Source: CAD feature listing. Evaluate the final solid. Frame: model axes, mm. Face numbers are marked on the shaded views. A direction names the side the tool comes from. Round coordinates to 2 decimals unless told otherwise and drop trailing zeros. Loops run counter-clockwise (first coordinate to the right, second up) from the corner with the lowest first, then second, coordinate; pieces in that order, holes last. Notation, with made-up numbers: (5.5, 7.25) -> (9.5, 7.25) arc R16 cw to (9.5, 33.25) -> close; hole circle Ø8 at (28, 75.25). An arc over 180 degrees is marked (long way). Write item = value, one per line.
from build123d import *

# Parameters (mm, degrees)
F0_R     = 20.6375
F0_R_2   = 6
F1_DEPTH = 237.33125
F2_DEPTH = 263.525
F3_R     = 3.175
F4_DEPTH = 6.35


with BuildPart() as f1:
    # F0 (on Right) → F1 (new body, symmetric)
    with BuildSketch(Plane.YZ):
        Circle(F0_R)
        Circle(F0_R_2, mode=Mode.SUBTRACT)
    extrude(amount=F1_DEPTH, both=True)

    # F0 (on Right) → F2 (join, symmetric)
    with BuildSketch(Plane.YZ):
        Circle(F0_R_2)
    extrude(amount=F2_DEPTH, both=True)

    # F3 (on Top) → F4 (cut, symmetric)
    with BuildSketch(Plane.XY):
        with Locations((255.5875, 0)):
            Circle(F3_R)
        with Locations((-255.5875, 0)):
            Circle(F3_R)
    extrude(amount=F4_DEPTH, both=True, mode=Mode.SUBTRACT)


solid = f1.part
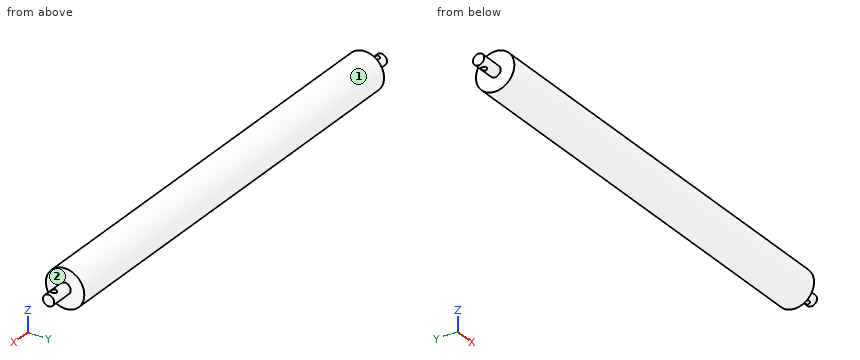
1. Section query C-C (z = -15.5). Return the cut outline in (x, y).
Evaluation:
outline = (-237.33, -13.63) -> (237.33, -13.63) -> (237.33, 13.63) -> (-237.33, 13.63) -> close
2. Contact query for flat-ended pins moving along their axis: pin 1 Ø4 at (y, z) = (-12.5, 0) entering from +X; pin 2 Ø8.5 at (x, y) = (-255.59, 0) entering from -Z; pin 3 Ø12 at (x, y) = (155, -1) entering from +Z. Output: stop coordinate, or through.
Evaluation:
pin_1 = 237.33
pin_2 = -6
pin_3 = 20.64
3. Line query: probe 1 along X at (y, z) = (0, 3) (1 decimal); probe 2 along X at (y, z) = (3, -13); probe 3 along Z at (x, y) = (-210, -15.5). Output: solid intervals per line, ascending. Write a range as from..to.
Evaluation:
probe_1 = -263.5..-258.8, -252.4..252.4, 258.8..263.5
probe_2 = -237.33..237.33
probe_3 = -13.63..13.63
4. Section query A-A (x = 90.5). Return the cut outline in (y, z) (1 decimal).
Evaluation:
outline = circle Ø41.3 at (0, 0)
5. Section query B-B (y = 12). Return the cut outline in (x, z), then the cut area to 3 significant figures.
Evaluation:
outline = (-237.33, -16.79) -> (237.33, -16.79) -> (237.33, 16.79) -> (-237.33, 16.79) -> close
area = 15,900 mm²
6. Set-up query: the marked faces 1 and 2. Return all of +Z, -Z, +X, -X, +Y, -Y with unobstructed straight access to the full face (end or side cutting, diameter ignored); none if empty.
Evaluation:
face_1 = +X, -X
face_2 = +X
